Study the drawing (mm; zero at the part's minimum x, y, z) and answer. Give positions to 0.01 mm unless a question says otherwise; leave off trailing zeros. Order: outer loops, then holes, each group sorted by start corner. A loop starts at its lowest first (then second) coordinate and runs counter-clockwise, first axis right, second up. Notation, with made-up numbers: (-35, 63) - (-5, 63) arc R16 ccw to (-5, 82) - close; hole circle Ø7 at (79.5, 73.25). An arc over 180 degrees is marked (long way). Write each question's results on one line, items separated by ' | '. Start each with the question number.
Q1. Find the intervals of material crossed by line 1 along Y through (x, z) = (4, 5); line 2 along Z through (x, y) = (12, 0.5); line 3 along Y through (x, z) = (18.5, 2.5), in increasing order. Write a range as from..to.
Q2. Find section A-A on z = 5. Give the vertices of the cut face in (x, y), and give its area (3 significant figures).
Q3. For a pull along Y with two mould halves and no side action, classify the marked faces 1, 2, 3 and 4 as +Y half, -Y half, draft (parallel to the pull), parting line (faces both ways), or undercut.
Q4. Find section B-B on x = 4.5. Give the vertices of the cut face in (y, z), and give its area (3 significant figures).
Q5. Find section D-D on z = 3. Give the vertices of the cut face in (x, y).
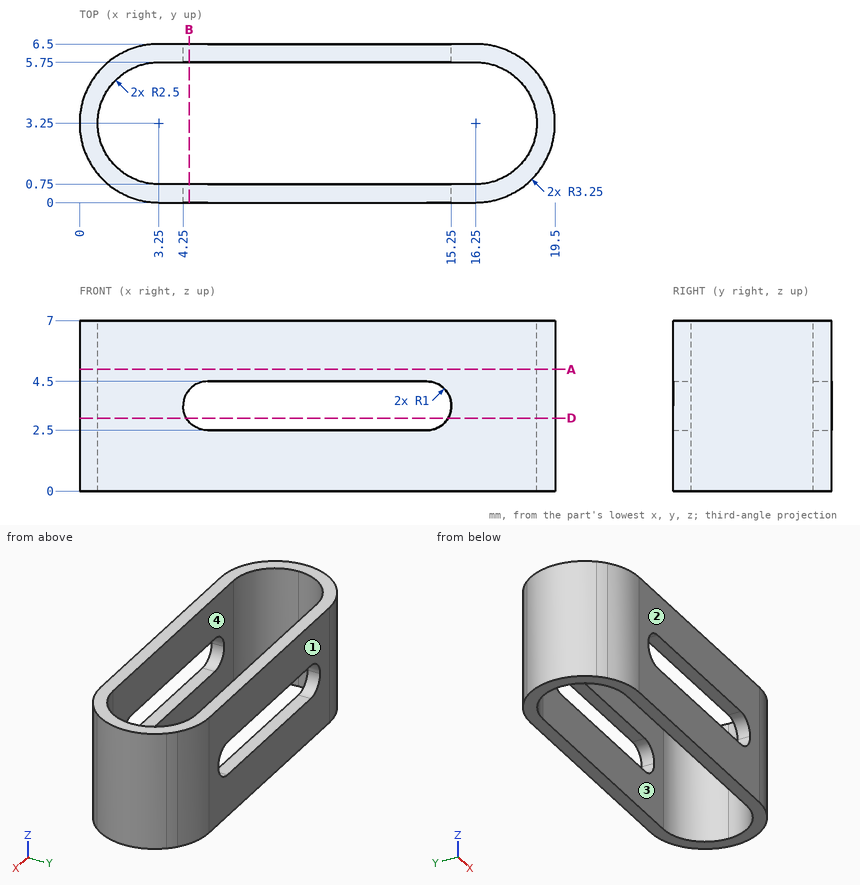
Working result:
1) line 1: 0..0.75, 5.75..6.5 | line 2: 0..2.5, 4.5..7 | line 3: 0.9..2.16, 4.34..5.6
2) outline: (3.25, 0) - (16.25, 0) arc R3.25 ccw to (16.25, 6.5) - (3.25, 6.5) arc R3.25 ccw to start; hole (3.25, 0.75) - (16.25, 0.75) arc R2.5 ccw to (16.25, 5.75) - (3.25, 5.75) arc R2.5 ccw to start | area: 33.0 mm²
3) face 1: +Y half | face 2: -Y half | face 3: undercut | face 4: undercut
4) outline: (0, 0) - (0.75, 0) - (0.75, 2.84) - (0, 2.84) - close; (0, 4.16) - (0.75, 4.16) - (0.75, 7) - (0, 7) - close; (5.75, 0) - (6.5, 0) - (6.5, 2.84) - (5.75, 2.84) - close; (5.75, 4.16) - (6.5, 4.16) - (6.5, 7) - (5.75, 7) - close | area: 8.52 mm²
5) outline: (3.25, 0) - (4.38, 0) - (4.38, 0.75) - (3.25, 0.75) arc R2.5 cw to (3.25, 5.75) - (4.38, 5.75) - (4.38, 6.5) - (3.25, 6.5) arc R3.25 ccw to start; (15.12, 0) - (16.25, 0) arc R3.25 ccw to (16.25, 6.5) - (15.12, 6.5) - (15.12, 5.75) - (16.25, 5.75) arc R2.5 cw to (16.25, 0.75) - (15.12, 0.75) - close
